from build123d import *

# Parameters (mm, degrees)
F0_W     = 63.5
F0_H     = 38.862
F0_H_2   = 26.162
F0_H_3   = 12.7
F1_DEPTH = 11.938
F2_W     = 13.97
F2_H     = 25.4
F3_DEPTH = 25.4
F4_W     = 63.5
F4_H     = 11.938
F5_DEPTH = 11.938


with BuildPart() as f1:
    # F0 (on Front) → F1 (new body)
    with BuildSketch(Plane.XZ):
        with BuildLine():
            Line((-70.517269, 199.179671), (-70.517269, 173.017671))
            Line((-70.517269, 173.017671), (-52.229269, 173.017671))
            ThreePointArc((-52.229269, 173.017671), (-38.767269, 186.479671), (-25.305269, 173.017671))
            Line((-25.305269, 173.017671), (-7.017269, 173.017671))
            Line((-7.017269, 173.017671), (-7.017269, 199.179671))
            Line((-7.017269, 199.179671), (-70.517269, 199.179671))
        make_face()
        with BuildLine():
            Line((-70.517269, 173.017671), (-70.517269, 134.155671))
            Line((-70.517269, 134.155671), (-52.229269, 134.155671))
            ThreePointArc((-52.229269, 134.155671), (-38.767269, 147.617671), (-25.305269, 134.155671))
            Line((-25.305269, 134.155671), (-7.017269, 134.155671))
            Line((-7.017269, 134.155671), (-7.017269, 173.017671))
            Line((-7.017269, 173.017671), (-25.305269, 173.017671))
            ThreePointArc((-25.305269, 173.017671), (-38.767269, 159.555671), (-52.229269, 173.017671))
            Line((-52.229269, 173.017671), (-70.517269, 173.017671))
        make_face()
        with BuildLine():
            Line((-70.517269, 134.155671), (-70.517269, 95.293671))
            Line((-70.517269, 95.293671), (-52.229269, 95.293671))
            ThreePointArc((-52.229269, 95.293671), (-38.767269, 108.755671), (-25.305269, 95.293671))
            Line((-25.305269, 95.293671), (-7.017269, 95.293671))
            Line((-7.017269, 95.293671), (-7.017269, 134.155671))
            Line((-7.017269, 134.155671), (-25.305269, 134.155671))
            ThreePointArc((-25.305269, 134.155671), (-38.767269, 120.693671), (-52.229269, 134.155671))
            Line((-52.229269, 134.155671), (-70.517269, 134.155671))
        make_face()
        with BuildLine():
            Line((-70.517269, 95.293671), (-70.517269, 64.051671))
            Line((-70.517269, 64.051671), (-52.229269, 64.051671))
            ThreePointArc((-52.229269, 64.051671), (-38.767269, 77.513671), (-25.305269, 64.051671))
            Line((-25.305269, 64.051671), (-7.017269, 64.051671))
            Line((-7.017269, 64.051671), (-7.017269, 95.293671))
            Line((-7.017269, 95.293671), (-25.305269, 95.293671))
            ThreePointArc((-25.305269, 95.293671), (-38.767269, 81.831671), (-52.229269, 95.293671))
            Line((-52.229269, 95.293671), (-70.517269, 95.293671))
        make_face()
        with BuildLine():
            Line((-70.517269, 64.051671), (-70.517269, 25.189671))
            Line((-70.517269, 25.189671), (-52.229269, 25.189671))
            ThreePointArc((-52.229269, 25.189671), (-38.767269, 38.651671), (-25.305269, 25.189671))
            Line((-25.305269, 25.189671), (-7.017269, 25.189671))
            Line((-7.017269, 25.189671), (-7.017269, 64.051671))
            Line((-7.017269, 64.051671), (-25.305269, 64.051671))
            ThreePointArc((-25.305269, 64.051671), (-38.767269, 50.589671), (-52.229269, 64.051671))
            Line((-52.229269, 64.051671), (-70.517269, 64.051671))
        make_face()
        with BuildLine():
            Line((-70.517269, 25.189671), (-70.517269, -13.672329))
            Line((-70.517269, -13.672329), (-52.229269, -13.672329))
            ThreePointArc((-52.229269, -13.672329), (-38.767269, -0.210329), (-25.305269, -13.672329))
            Line((-25.305269, -13.672329), (-7.017269, -13.672329))
            Line((-7.017269, -13.672329), (-7.017269, 25.189671))
            Line((-7.017269, 25.189671), (-25.305269, 25.189671))
            ThreePointArc((-25.305269, 25.189671), (-38.767269, 11.727671), (-52.229269, 25.189671))
            Line((-52.229269, 25.189671), (-70.517269, 25.189671))
        make_face()
        with BuildLine():
            Line((-70.517269, -13.672329), (-70.517269, -52.534329))
            Line((-70.517269, -52.534329), (-52.229269, -52.534329))
            ThreePointArc((-52.229269, -52.534329), (-38.767269, -39.072329), (-25.305269, -52.534329))
            Line((-25.305269, -52.534329), (-7.017269, -52.534329))
            Line((-7.017269, -52.534329), (-7.017269, -13.672329))
            Line((-7.017269, -13.672329), (-25.305269, -13.672329))
            ThreePointArc((-25.305269, -13.672329), (-38.767269, -27.134329), (-52.229269, -13.672329))
            Line((-52.229269, -13.672329), (-70.517269, -13.672329))
        make_face()
        with BuildLine():
            Line((-70.517269, -52.534329), (-70.517269, -91.396329))
            Line((-70.517269, -91.396329), (-52.229269, -91.396329))
            ThreePointArc((-52.229269, -91.396329), (-38.767269, -77.934329), (-25.305269, -91.396329))
            Line((-25.305269, -91.396329), (-7.017269, -91.396329))
            Line((-7.017269, -91.396329), (-7.017269, -52.534329))
            Line((-7.017269, -52.534329), (-25.305269, -52.534329))
            ThreePointArc((-25.305269, -52.534329), (-38.767269, -65.996329), (-52.229269, -52.534329))
            Line((-52.229269, -52.534329), (-70.517269, -52.534329))
        make_face()
        with BuildLine():
            Line((-70.517269, -91.396329), (-70.517269, -130.258329))
            Line((-70.517269, -130.258329), (-7.017269, -130.258329))
            Line((-7.017269, -130.258329), (-7.017269, -91.396329))
            Line((-7.017269, -91.396329), (-25.305269, -91.396329))
            ThreePointArc((-25.305269, -91.396329), (-38.767269, -104.858329), (-52.229269, -91.396329))
            Line((-52.229269, -91.396329), (-70.517269, -91.396329))
        make_face()
        with Locations((-38.767269, -149.689329)):
            Rectangle(F0_W, F0_H)
        with Locations((-38.767269, -182.201329)):
            Rectangle(F0_W, F0_H_2)
        with Locations((-38.767269, -201.632329)):
            Rectangle(F0_W, F0_H_3)
    extrude(amount=F1_DEPTH)

    # F2 (on face) → F3 (cut)
    with BuildSketch(Plane(origin=(0, 0, 0), x_dir=(-1, 0, 0), z_dir=(0, 1, 0))):
        with Locations((38.767269, -169.120329)):
            Rectangle(F2_W, F2_H)
    extrude(amount=-F3_DEPTH, mode=Mode.SUBTRACT)

    # F4 (on face) → F5 (join)
    with BuildSketch(Plane(origin=(0, 0, -207.982329), x_dir=(1, 0, 0), z_dir=(0, 0, -1))):
        with Locations((-38.767269, 5.969)):
            Rectangle(F4_W, F4_H)
    extrude(amount=F5_DEPTH)


solid = f1.part
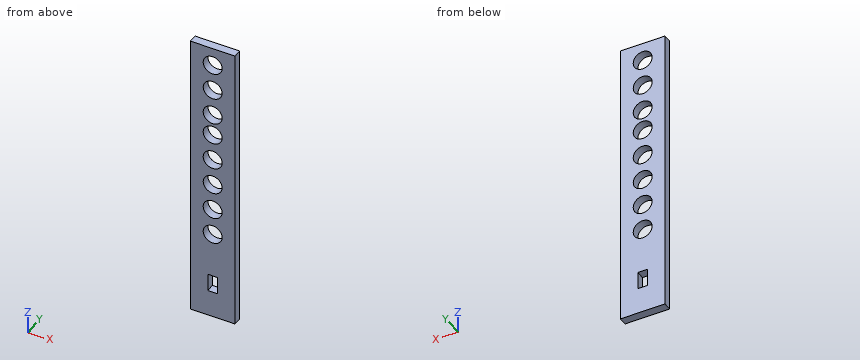
Source: CAD feature listing. Evaluate the final solid. Frame: model axes, mm. Give positions to 0.01 mm unless a question says otherwise; leave off trailing zeros. Write each loop counter-clockwise with the first axis right and the second up, starting at its lowest first coordinate (ties: lowest second). Pieces come first, ordered by that corner, then holes. Notation, with made-up numbers: (17.5, 12) -> (25.5, 12) arc R9 cw to (25.5, 23) -> close; hole circle Ø8 at (50, 40.5). An arc over 180 degrees is marked (long way). Write item = value, one per line.
Q1. Cut plane D-D on z = -58. Return loops of the section in (x, y), then the cut area to 3 significant figures.
Here are the results:
outline = (-70.52, -11.94) -> (-51.07, -11.94) -> (-51.07, 0) -> (-70.52, 0) -> close; (-26.46, -11.94) -> (-7.02, -11.94) -> (-7.02, 0) -> (-26.46, 0) -> close
area = 464 mm²
Q2. Line query: line 1 (X direction, y = -8, z = 133.5); line 2 (X direction, y = -5.25, z = 128.5). Output: solid intervals per line, ascending. Write a range as from..to.
Here are the results:
line_1 = -70.52..-52.21, -25.32..-7.02
line_2 = -70.52..-50.98, -26.55..-7.02
Q3. Cut plane B-B on y = -4. State how many separate pieces and enclosed holes the cut face has, then the cut area to 3 significant figures.
Here are the results:
separate_pieces = 1
enclosed_holes = 9
area = 21,700 mm²
Q4. First-contact query: pin 1 (3 mm diameter, centred on x = -16, z = -50, fed in from +Y). Flat tip, straight axial feed; report the tip coordinate or a pass-through.
Here are the results:
pin_1 = 0
Q5. Cut plane A-A on z = -163. Return loops of the section in (x, y), then the cut area to 3 significant figures.
Here are the results:
outline = (-70.52, -11.94) -> (-45.75, -11.94) -> (-45.75, 0) -> (-70.52, 0) -> close; (-31.78, -11.94) -> (-7.02, -11.94) -> (-7.02, 0) -> (-31.78, 0) -> close
area = 591 mm²
